Check sheet for the modelled part. Datum: model origin and axes. Units: mm. A direction names the side the tool comes from. Round coordinates to 2 decimals unless told otherwise and drop trailing zeros. Order: outer loops, then holes, each group sorted by start corner. A loop starts at its lowest first (then second) coordinate and runs counter-clockwise, first axis right, second up.
```python
from build123d import *

# Parameters (mm, degrees)
CROQUIS1_R              = 14
SALIENTE_EXTRUIR1_DEPTH = 18
CROQUIS2_R              = 2.5
SALIENTE_EXTRUIR3_DEPTH = 2
SALIENTE_EXTRUIR4_DEPTH = 2
SALIENTE_EXTRUIR5_DEPTH = 6


with BuildPart() as part:
    # Croquis1 → Saliente-Extruir1 (new body)
    with BuildSketch(Plane.XY):
        Circle(CROQUIS1_R)
        with BuildLine():
            ThreePointArc((7, -12.124355653), (3.623466631, -13.522961568), (0, -14))
            Line((0, -14), (0, -16))
            Line((0, -16), (7, -16))
            Line((7, -16), (7, -12.124355653))
        make_face()
        with BuildLine():
            Line((0, -16), (0, -14))
            ThreePointArc((0, -14), (-3.623466631, -13.522961568), (-7, -12.124355653))
            Line((-7, -12.124355653), (-7, -16))
            Line((-7, -16), (0, -16))
        make_face()
    extrude(amount=SALIENTE_EXTRUIR1_DEPTH)

    # Croquis2 → Saliente-Extruir3 (add)
    # profile 1 of 2: a face of its own
    with BuildSketch(Plane(origin=(0, 0, 0), x_dir=(-1, 0, 0), z_dir=(0, 0, -1))):
        with BuildLine():
            Line((-17.5, 4.5), (-13.257073584, 4.5))
            ThreePointArc((-13.257073584, 4.5), (-14, 0), (-13.257073584, -4.5))
            Line((-13.257073584, -4.5), (-17.5, -4.5))
            ThreePointArc((-17.5, -4.5), (-22, 0), (-17.5, 4.5))
        make_face()
        with Locations((-17.5, 0)):
            Circle(CROQUIS2_R, mode=Mode.SUBTRACT)
    # profile 2 of 2: a face of its own
    with BuildSketch(Plane(origin=(0, 0, 0), x_dir=(-1, 0, 0), z_dir=(0, 0, -1))):
        with BuildLine():
            Line((17.5, -4.5), (13.257073584, -4.5))
            ThreePointArc((13.257073584, -4.5), (14, 0), (13.257073584, 4.5))
            Line((13.257073584, 4.5), (17.5, 4.5))
            ThreePointArc((17.5, 4.5), (22, 0), (17.5, -4.5))
        make_face()
        with Locations((17.5, 0)):
            Circle(CROQUIS2_R, mode=Mode.SUBTRACT)
    extrude(amount=-SALIENTE_EXTRUIR3_DEPTH)

    # Croquis3 → Saliente-Extruir4 (add)
    with BuildSketch(Plane(origin=(0, 0, 0), x_dir=(-1, 0, 0), z_dir=(0, 0, -1))):
        with BuildLine():
            ThreePointArc((4, 9), (2.828427125, 11.828427125), (0, 13))
            Line((0, 13), (0, 5))
            ThreePointArc((0, 5), (2.828427125, 6.171572875), (4, 9))
        make_face()
        with BuildLine():
            Line((0, 5), (0, 13))
            ThreePointArc((0, 13), (-4, 9), (0, 5))
        make_face()
    extrude(amount=SALIENTE_EXTRUIR4_DEPTH)

    # Croquis4 → Saliente-Extruir5 (add)
    with BuildSketch(Plane(origin=(0, 0, -2), x_dir=(-1, 0, 0), z_dir=(0, 0, -1))):
        with BuildLine():
            ThreePointArc((1.5612495, 10.25), (0, 11), (-1.5612495, 10.25))
            Line((-1.5612495, 10.25), (-1.5612495, 7.75))
            ThreePointArc((-1.5612495, 7.75), (0, 7), (1.5612495, 7.75))
            Line((1.5612495, 7.75), (1.5612495, 10.25))
        make_face()
    extrude(amount=SALIENTE_EXTRUIR5_DEPTH)


solid = part.part
```
Item 1: Sectioned sample at D-D (y = -12.75). Record the cut outline in (x, z), and give its area (3 significant figures).
Answer:
outline: (-7, 0) - (7, 0) - (7, 18) - (-7, 18) - close
area: 252 mm2
Item 2: Sectioned sample at C-C (z = 10). Record the cut outline in (x, y), and give its area (3 significant figures).
Answer:
outline: (-7, -16) - (7, -16) - (7, -12.12) arc R14 ccw (long way) to (-7, -12.12) - close
area: 652 mm2
Item 3: Scan lines: line 1 along Y through (x, z) = (-17.5, 1.45); line 2 along Z through (x, y) = (6, -8.75); line 3 along Z through (x, y) = (15, 2). Record each from-to range of solid material in increasing order.
Answer:
line 1: y = -4.5 to -2.5, 2.5 to 4.5
line 2: z = 0 to 18
line 3: z = 0 to 2
Item 4: Release check for a two-part mould opening along X. For faces 5 (the cylindrical face through (22, 0, 1)), 6 (the flat face through (0, -16, 9)), 7 (the cylindrical face through (20, 0, 1)) record: released by +X, released by -X, zero draft, split by the parting line, or undercut.
Answer:
face 5: released by +X
face 6: zero draft
face 7: undercut
Item 5: Sectioned sample at B-B (x = 2.5). Record the cut outline in (y, z).
Answer:
outline: (-16, 0) - (5.88, 0) - (5.88, -2) - (12.12, -2) - (12.12, 0) - (13.77, 0) - (13.77, 18) - (-16, 18) - close
Item 6: Sectioned sample at A-A (y = 0). Record the cut outline in (x, z).
Answer:
outline: (-22, 0) - (-20, 0) - (-20, 2) - (-22, 2) - close; (-15, 0) - (15, 0) - (15, 2) - (14, 2) - (14, 18) - (-14, 18) - (-14, 2) - (-15, 2) - close; (20, 0) - (22, 0) - (22, 2) - (20, 2) - close
Item 7: Access from +Z, -Z, +X, -X, +Y, -Y to the whole of each face (thin tool, end or side, straight path). Record for faces 1 (the cylindrical face through (0, 11, -5)), 2 (the flat face through (15, -4.5, 1)), 3 (the cylindrical face through (0, 7, -5)), 4 (the flat face through (-15, 4.5, 1)).
Answer:
face 1: -Z, +Y
face 2: +Z, -Z, +X, -Y
face 3: -Z, -Y
face 4: +Z, -Z, -X, +Y
Item 8: Go/stop test with flat-tipped pins: P1, Ø3, axis at y = 9, z = -4, coming from the -X side; P2, Ø1.2, axis at y = -13, z = 7, coming from the -X side; P3, Ø3, axis at x = 17.5, y = 0, coming from the +Z side; P4, Ø5, axis at x = -3, y = -9.5, coming from the -Z side. Record where each tip stops, or that it passes through.
Answer:
P1: stops at x = -1.56
P2: stops at x = -7
P3: passes through
P4: stops at z = 0
